Part model, mm, in its own coordinate system. A direction names the side the tool comes from. Round coordinates to 2 decimals unless told otherwise and drop trailing zeros. Write each loop counter-clockwise with the first axis right and the second up, starting at its lowest first coordinate (ties: lowest second). Pieces come first, ordered by that corner, then holes. Notation, with made-up numbers: (-19, -13) -> (40, -13) arc R29 ccw to (40, 19) -> close; hole circle Ø11 at (64.25, 8.5). An arc over 180 degrees is marked (long way). Use CSV: the item, a comma, the result in double quotes. Start each with the question number.
(1) Saw through at B-B (x = -10). Give the cut face in (y, z).
(2) Two-plate mould, pull along X, no slides. Class faces 6 (the flat face through (-33, 0, 30)), 7 (the flat face through (27, -15, 6)), 8 (the flat face through (0, 0, 0)), 9 (the flat face through (-21, 0, 36)): released by +X, released by -X, zero draft, split by the parting line, or undercut.
(3) Saw through at D-D (y = -3). Give the cut face in (x, z), plus the area to 3 significant figures.
(4) Drop flat-ended pins along their axis: pin 1 (1.5 mm diameter, centred on y = 2.5, z = 28, fed in from +X); pin 2 (21 mm diameter, centred on x = 10.5, z = 34, fed in from -Y); pin 3 (1 mm diameter, centred on y = 3, z = 32.5, fed in from +X); pin 4 (5 mm diameter, centred on x = -25.5, z = 40.5, fed in from +Y). Give the stop position or say it passes through.
(5) Saw through at A-A (z = 50). Give the cut face in (x, y).
(6) Which spindle directions (+Z, -Z, +X, -X, +Y, -Y) get a long thin tool onto all of the face, cutting with end or side? Do faces 1 (the flat face through (-20.609, 0, 33)), 2 (the cylindrical face through (-27.1, 14.7, 54)), 3 (the flat face through (-12, -21, 11)), 4 (the flat face through (0, -6, 28)), 5 (the flat face through (0, 6, 28)). Say none if no direction does.
(7) Saw through at C-C (z = 9.5). Give the cut face in (x, y).
(8) Probe line 1 (Y direction, x = 12, z = 22); line 2 (Z direction, x = -17, y = -16.5); line 3 (X direction, y = -10.5, z = 23.5). List the from-to ranges inside material, lowest first. Write a range as [from, to].
Autodesk Fusion 360 part; units mm, degrees
sketch "bottom" plane through (0, 0, 0) normal (0, 0, 1) x (1, 0, 0)
  line L0 (33, 21) -> (-33, 21)
  line L1 (-33, 21) -> (-33, -21)
  line L2 (-33, -21) -> (33, -21)
  line L3 (33, -21) -> (33, 21)
  line L4 (33, 21) -> (-33, -21) construction
  line L5 (-33, 21) -> (33, -21) construction
  dimension "d1" = 66
  dimension "d2" = 42
extrude "Extrude1" add sketch "bottom" along normal blind 12
chamfer "Chamfer1" distance 12 angle 45 2 edges at (33, -21, 6) (33, 21, 6)
sketch "vertical" plane through (0, 0, 12) normal (0, 0, 1) x (-1, 0, 0)
  line L0 (-33, -9) -> (-21, -21)
  line L1 (-21, -21) -> (33, -21)
  line L2 (33, -21) -> (33, 21)
  line L3 (33, 21) -> (-21, 21)
  line L4 (-21, 21) -> (-33, 9)
  line L5 (-33, 9) -> (-33, -9)
  line L6 (33, -21) -> (21, -21)
  line L7 (21, -21) -> (21, 21)
  line L8 (21, 21) -> (33, 21)
  line L9 (33, 21) -> (33, -21)
  dimension "d6" = 12
extrude "Extrude2" add sketch "vertical" along normal blind 48 contours L1 L2 L3 L6 L7 L8 L9
fillet "Fillet1" radius 21 2 edges at (-27, -21, 60) (-27, 21, 60)
sketch "triangle" plane through (0, 0, 0) normal (0, 1, 0) x (1, 0, 0)
  line L0 (-20.6092, -11.7383) -> (-20.6092, -53.7383)
  line L1 (-20.6092, -53.7383) -> (33, -12)
  line L2 (33, -12) -> (-20.6092, -11.7383)
  dimension "d10" = 42
extrude "Extrude4" add sketch "triangle" along normal mid plane 12
extrude "Extrude3" [suppressed]
Answers:
1,outline,"(-21, 0) -> (21, 0) -> (21, 12) -> (6, 12) -> (6, 45.48) -> (-6, 45.48) -> (-6, 12) -> (-21, 12) -> close"
2,face 6,"released by -X"
2,face 7,"released by +X"
2,face 8,"zero draft"
2,face 9,"undercut"
3,outline,"(-33, 0) -> (33, 0) -> (33, 12) -> (-20.61, 53.74) -> (-20.61, 12) -> (-21, 12) -> (-21, 59.79) -> (-33, 59.79) -> close"
3,area,"2,480 mm²"
4,pin 1,"stops at x = 13.41"
4,pin 2,"stops at y = -6"
4,pin 3,"stops at x = 7.31"
4,pin 4,"stops at y = 21"
5,outline,"(-33, -17.89) -> (-21, -17.89) -> (-21, 17.89) -> (-33, 17.89) -> close; (-20.61, -6) -> (-15.81, -6) -> (-15.81, 6) -> (-20.61, 6) -> close"
6,face 1,"+Z, +Y, -Y"
6,face 2,"+Z, +X, -X, +Y"
6,face 3,"+Z, -Z, +X, -X, -Y"
6,face 4,"+Z, +X, -Y"
6,face 5,"+Z, +X, +Y"
7,outline,"(-33, -21) -> (21, -21) -> (33, -9) -> (33, 9) -> (21, 21) -> (-33, 21) -> close"
8,line 1,"y = [-6, 6]"
8,line 2,"z = [0, 12]"
8,line 3,"x = [-33, -21]"
